from build123d import *

# Parameters (mm, degrees)
SKETCH_1_R               = 45
EXTRUDE_1_DEPTH          = 4
SKETCH_2_R               = 2.15
CUT_EXTRUDE_1_DEPTH      = 64.765194268
PATTERN_CIRCULAR_1_COUNT = 6
CUT_EXTRUDE_2_DEPTH      = 64.765194268
CUT_EXTRUDE_2_DEPTH_BACK = 64.765194268
SKETCH_3_R               = 8.5
SKETCH_4_R               = 1.65
CUT_EXTRUDE_3_DEPTH      = 64.765194268
PATTERN_CIRCULAR_2_COUNT = 8
SKETCH_5_R               = 17.6
CUT_EXTRUDE_4_DEPTH      = 1.2
SKETCH_6_R               = 1.975
CUT_EXTRUDE_5_DEPTH      = 64.765194268
PATTERN_CIRCULAR_3_COUNT = 8


with BuildPart() as part:
    # 草图1 → 凸台-拉伸1 (new body)
    with BuildSketch(Plane(origin=(0, 0, 0), x_dir=(1, 0, 0), z_dir=(0, 1, 0))):
        with Locations(Location((0, 0, 0), (0, 0, 270))):
            Circle(SKETCH_1_R)
    extrude(amount=EXTRUDE_1_DEPTH)

    # 草图2 → 切除-拉伸1 (cut, symmetric)
    with BuildSketch(Plane(origin=(0, 4, 0), x_dir=(1, 0, 0), z_dir=(0, 1, 0))):
        with Locations(Location((0, 14, 0), (0, 0, 270))):
            Circle(SKETCH_2_R)
    cut_extrude_1 = extrude(amount=CUT_EXTRUDE_1_DEPTH, both=True, mode=Mode.SUBTRACT)

    # 阵列(圆周)1: 切除-拉伸1 ×6 about axis
    pattern_circular_1_axis = Axis((0, 0, 0), (0, 1, 0))
    for i in range(1, PATTERN_CIRCULAR_1_COUNT):
        add(cut_extrude_1.rotate(pattern_circular_1_axis, i * 360 / PATTERN_CIRCULAR_1_COUNT), mode=Mode.SUBTRACT)

    # 草图3 → 切除-拉伸2 (cut, two sides: drawn at the far end of the back side and taken through both)
    with BuildSketch(Plane(origin=(0, 4, 0), x_dir=(1, 0, 0), z_dir=(0, 1, 0)).offset(-CUT_EXTRUDE_2_DEPTH_BACK)):
        with Locations(Location((0, 0, 0), (0, 0, 270))):
            Circle(SKETCH_3_R)
    extrude(amount=CUT_EXTRUDE_2_DEPTH + CUT_EXTRUDE_2_DEPTH_BACK, mode=Mode.SUBTRACT)

    # 草图4 → 切除-拉伸3 (cut, symmetric)
    with BuildSketch(Plane(origin=(0, 4, 0), x_dir=(1, 0, 0), z_dir=(0, 1, 0))):
        with Locations(Location((0, 37, 0), (0, 0, 270))):
            Circle(SKETCH_4_R)
    cut_extrude_3 = extrude(amount=CUT_EXTRUDE_3_DEPTH, both=True, mode=Mode.SUBTRACT)

    # 阵列(圆周)2: 切除-拉伸3 ×8 about axis
    pattern_circular_2_axis = Axis((0, 0, 0), (0, 1, 0))
    for i in range(1, PATTERN_CIRCULAR_2_COUNT):
        add(cut_extrude_3.rotate(pattern_circular_2_axis, i * 360 / PATTERN_CIRCULAR_2_COUNT), mode=Mode.SUBTRACT)

    # 草图5 → 切除-拉伸4 (cut)
    with BuildSketch(Plane.XZ):
        with Locations(Location((0, 0, 0), (0, 0, 270))):
            Circle(SKETCH_5_R)
    extrude(amount=-CUT_EXTRUDE_4_DEPTH, mode=Mode.SUBTRACT)

    # 草图6 → 切除-拉伸5 (cut, symmetric)
    with BuildSketch(Plane(origin=(0, 4, 0), x_dir=(1, 0, 0), z_dir=(0, 1, 0))):
        with Locations(Location((14.551537516, -35.130519224, 0), (0, 0, 270))):
            Circle(SKETCH_6_R)
    cut_extrude_5 = extrude(amount=CUT_EXTRUDE_5_DEPTH, both=True, mode=Mode.SUBTRACT)

    # 阵列(圆周)3: 切除-拉伸5 ×8 about axis
    pattern_circular_3_axis = Axis((0, 0, 0), (0, 1, 0))
    for i in range(1, PATTERN_CIRCULAR_3_COUNT):
        add(cut_extrude_5.rotate(pattern_circular_3_axis, i * 360 / PATTERN_CIRCULAR_3_COUNT), mode=Mode.SUBTRACT)


solid = part.part
For this review, take the finished solid that the model builds, in its own axes (mm). Coordinates: 2 decimals unless noted, no trailing zeros. Write each loop counter-clockwise with the first axis right and the second up, starting at its lowest first coordinate (ties: lowest second). Pieces come first, ordered by that corner, then holes. Notation, with made-up numbers: (-9, 87.25) -> (34, 87.25) arc R16 cw to (34, 94.25) -> close; hole circle Ø10 at (17, -23). An arc over 180 degrees is marked (long way). Write each question's results on one line, items separated by ' | '. Start each with the question number.
1) Insertion check: pin 1 (17.5 mm diameter, centred on x = -4, z = -2.5, fed in from -Y); pin 2 (1 mm diameter, centred on y = 3, z = 33.5, fed in from +X); pin 3 (1.5 mm diameter, centred on x = 13.5, y = 3.5, fed in from +Z). Each pin has a flat end and moves straight along its axis. Give the tip position at first contact, or say it passes through.
2) The part is to be moulded in two halves that separate along X. For faces 1 (the face through (25.53, 2.03, 24.64)), 2 (the face through (-9, 4, -1)), 3 (the face through (-17.235, 1.972, 41.569)), say which applies: +X half, -X half, draft (parallel to the pull), parting line (faces both ways), or undercut.
3) Consider section D-D (x = 21). Write out the cut boundary in (y, z).
4) Consider section A-A (z = 0). Write out the cut boundary in (x, y).
5) Wall thickness on L1, parallel to X at y = 2.9, z = -25.5; L2, parallel to X at y = 2.8, z = 14.5; L3, parallel to Z at x = -13.5, y = 3.35: over which ranges is each line inside the solid? List them lowest first. Write a range as [from, to].
6) Consider section B-B (y = 2.35). Give the number of separate pieces and of enclosed holes in the cut face, plus the area to 3 significant figures.
7) Consider section C-C (z = -32). Write out the cut boundary in (x, y).
Geometry says:
1) pin 1: y = 1.2 | pin 2: x = 30.59 | pin 3: z = 43.16
2) face 1: undercut | face 2: draft | face 3: parting line
3) outline: (0, -39.8) -> (4, -39.8) -> (4, 39.8) -> (0, 39.8) -> close
4) outline: (-45, 0) -> (-38.65, 0) -> (-38.65, 4) -> (-45, 4) -> close; (-35.35, 0) -> (-17.6, 0) -> (-17.6, 1.2) -> (-8.5, 1.2) -> (-8.5, 4) -> (-35.35, 4) -> close; (8.5, 1.2) -> (17.6, 1.2) -> (17.6, 0) -> (35.35, 0) -> (35.35, 4) -> (8.5, 4) -> close; (38.65, 0) -> (45, 0) -> (45, 4) -> (38.65, 4) -> close
5) L1: [-37.08, -27.67], [-24.65, 24.65], [27.67, 37.08] | L2: [-42.6, -37.1], [-33.16, -2.09], [2.09, 33.16], [37.1, 42.6] | L3: [-42.93, -36.8], [-33.46, -8.65], [-5.35, 5.35], [8.65, 33.46], [36.8, 42.93]
6) separate pieces: 1 | enclosed holes: 23 | area: 5,880 mm^2
7) outline: (-31.64, 0) -> (31.64, 0) -> (31.64, 4) -> (-31.64, 4) -> close
